```python
from build123d import *

# Parameters (mm, degrees)
SKETCH_1_W                 = 5.6
SKETCH_1_H                 = 4.2
EXTRUDE_1_DEPTH            = 1.4
SKETCH_3_W                 = 25.5
SKETCH_3_H                 = 0.3
SKETCH_3_W_2               = 5.6
EXTRUDE_2_DEPTH            = 0.2
PATTERN_START              = -2.1
PATTERN_LINEAR_1_OUTLINE_W = 5.6
PATTERN_LINEAR_1_OUTLINE_H = 1.4
PATTERN_LINEAR_1_DEPTH     = 4.2
SKETCH_4_W                 = 2.9
SKETCH_4_H                 = 1.1
SKETCH_4_H_2               = 0.55
CUT_EXTRUDE_1_DEPTH        = 0.2
SKETCH_5_W                 = 0.2
SKETCH_5_H                 = 0.8
EXTRUDE_3_DEPTH            = 0.8
SKETCH_6_W                 = 0.2
SKETCH_6_H                 = 0.8
EXTRUDE_4_DEPTH            = 0.8
SKETCH_7_W                 = 32.884134448
SKETCH_7_H                 = 1
EXTRUDE_5_DEPTH            = 0.2
CUT_EXTRUDE_START          = -0.4
SKETCH_8_W                 = 4.4
SKETCH_8_H                 = 3
CUT_EXTRUDE_2_DEPTH        = 1


# Read off the part's stored shape, not the designer's step: the pattern linear step
with BuildPart() as part:
    # Sketch 1 → Extrude 1 (new body)
    with BuildSketch(Plane.XY):
        Rectangle(SKETCH_1_W, SKETCH_1_H)
    extrude(amount=EXTRUDE_1_DEPTH)

    # Sketch 3 → Extrude 2 (add)
    with BuildSketch(Plane(origin=(0, 0, 0), x_dir=(-1, 0, 0), z_dir=(0, 0, -1))):
        Polygon((-2.8, 2.1), (2.8, 2.1), (2.8, 3.3), (-28.3, 3.3), (-28.3, 2.1), align=None)
        with Locations((-15.55, 1.95)):
            Rectangle(SKETCH_3_W, SKETCH_3_H)
        with Locations((0, 1.95)):
            Rectangle(SKETCH_3_W_2, SKETCH_3_H)
    extrude(amount=-EXTRUDE_2_DEPTH)

    # Pattern Linear 1 outline → Pattern Linear 1 (add)
    with BuildSketch(Plane(origin=(0, 0, 0), x_dir=(1, 0, 0), z_dir=(0, 1, 0)).offset(PATTERN_START)):
        with Locations((8.5, -0.7)):
            Rectangle(PATTERN_LINEAR_1_OUTLINE_W, PATTERN_LINEAR_1_OUTLINE_H)
        with Locations((17, -0.7)):
            Rectangle(PATTERN_LINEAR_1_OUTLINE_W, PATTERN_LINEAR_1_OUTLINE_H)
        with Locations((25.5, -0.7)):
            Rectangle(PATTERN_LINEAR_1_OUTLINE_W, PATTERN_LINEAR_1_OUTLINE_H)
    extrude(amount=PATTERN_LINEAR_1_DEPTH)

    # Sketch 4 → Cut-Extrude 1 (cut)
    with BuildSketch(Plane(origin=(0, 0, 0), x_dir=(-1, 0, 0), z_dir=(0, 0, -1))):
        with Locations((-4.25, 1.8)):
            Rectangle(SKETCH_4_W, SKETCH_4_H)
        with Locations((-12.75, 1.8)):
            Rectangle(SKETCH_4_W, SKETCH_4_H)
        with Locations((-21.25, 1.525)):
            Rectangle(SKETCH_4_W, SKETCH_4_H_2)
        with Locations((-21.25, 2.075)):
            Rectangle(SKETCH_4_W, SKETCH_4_H_2)
    extrude(amount=-CUT_EXTRUDE_1_DEPTH, mode=Mode.SUBTRACT)

    # Sketch 5 → Extrude 3 (add)
    with BuildSketch(Plane(origin=(28.3, 0, 0), x_dir=(0, 0, -1), z_dir=(1, 0, 0))):
        with Locations((-0.1, 2.9)):
            Rectangle(SKETCH_5_W, SKETCH_5_H)
    extrude(amount=EXTRUDE_3_DEPTH)

    # Sketch 6 → Extrude 4 (add)
    with BuildSketch(Plane.ZY.offset(2.8)):
        with Locations((0.1, 2.9)):
            Rectangle(SKETCH_6_W, SKETCH_6_H)
    extrude(amount=EXTRUDE_4_DEPTH)

    # Sketch 7 → Extrude 5 (add)
    with BuildSketch(Plane(origin=(0, 0, 0), x_dir=(-1, 0, 0), z_dir=(0, 0, -1))):
        with Locations((-12.798406479, -1.6)):
            Rectangle(SKETCH_7_W, SKETCH_7_H)
    extrude(amount=-EXTRUDE_5_DEPTH)

    # Sketch 8 → Cut-Extrude 2 (cut)
    with BuildSketch(Plane.XY.offset(1.4).offset(CUT_EXTRUDE_START)):
        Rectangle(SKETCH_8_W, SKETCH_8_H)
        with Locations((8.5, 0)):
            Rectangle(SKETCH_8_W, SKETCH_8_H)
        with Locations((17, 0)):
            Rectangle(SKETCH_8_W, SKETCH_8_H)
        with Locations((25.5, 0)):
            Rectangle(SKETCH_8_W, SKETCH_8_H)
    extrude(amount=-CUT_EXTRUDE_2_DEPTH, mode=Mode.SUBTRACT)


solid = part.part
```
Source: CAD feature listing. Evaluate the final solid. Frame: model axes, mm. A direction names the side the tool comes from. Coordinates: 2 decimals unless noted, no trailing zeros. Loops run counter-clockwise (first coordinate to the right, second up) from the corner with the lowest first, then second, coordinate; pieces in that order, holes last. Notation, with made-up numbers: M -27.75,46 L 10.25,46 A15 cw 10.25,66 Z; hole C 76.25,39 d5. An arc over 180 degrees is marked long. Put each result on its own line as item: value. Start each with the question number.
1) Cut plane C-C on x = 5. Return the cut outline in (y, z), then the cut area to 3 significant figures.
2) Cut plane D-D on x = 25.5. Return the cut outline in (y, z), then the cut area to 3 significant figures.
3) Ray query, L1, parallel to X at y = 2.2, z = 0.15; L2, parallel to Y at x = 24.5, z = 0.35; L3, parallel to Y at x = -2, z = 0.15. Return the intervals inside material, ascending. Write a range as from..to.
4) Reachability of faces 4 (the face through (17, 1.5, 0.5)), 5 (the face through (25, 0, 1.4)), 6 (the face through (-3.2, -1.6, 0.2)), 7 (the face through (0, 2.1, 1)) from +Z, -Z, +X, -X, +Y, -Y: full face, straight path, thin tool, end or side. Return the list, or none.
5) Cut plane A-A on y = 0.8. Give the number of separate pieces and of enclosed holes in the cut face, then the cut area to 3 significant figures.
6) Pull-direction query (X, two-part tool) for faces 1 (the face through (2.8, 0, 1)), 2 (the face through (17, 2.1, 1)), 3 (the face through (17, 0, 1)); classes: pulls with the +X half, pulls with the -X half, needs draft (parallel to the pull), parting line crosses it, or undercut.
7) Contact query for flat-ended pins moving along their axis: pin 1 Ø0.5 at (x, y) = (21, -1.5) entering from +Z; pin 2 Ø0.7 at (y, z) = (0, 1) entering from -X; pin 3 Ø0.7 at (y, z) = (1, 0.5) entering from +X; pin 4 Ø0.8 at (x, y) = (28.5, -1.5) entering from +Z. Output: stop coordinate, or through.
The answers:
1. outline: M -2.1,0 L -1.1,0 L -1.1,0.2 L -2.1,0.2 Z; M 2.35,0 L 3.3,0 L 3.3,0.2 L 2.35,0.2 Z
1. area: 0.390 mm²
2. outline: M -2.1,0 L -1.5,0 L -1.5,1 L 1.5,1 L 1.5,0 L 3.3,0 L 3.3,0.2 L 2.1,0.2 L 2.1,1.4 L -2.1,1.4 Z
2. area: 3.12 mm²
3. L1: x = -2.8..2.8, 5.7..11.3, 14.2..19.8, 22.7..28.3
3. L2: y = -2.1..-1.5, 1.5..2.1
3. L3: y = -2.1..-1.5, 1.5..3.3
4. face 4: -Z
4. face 5: +Z, +X, -X, +Y, -Y
4. face 6: +Z, -X, +Y, -Y
4. face 7: +Z, +X, -X, +Y
5. separate pieces: 4
5. enclosed holes: 0
5. area: 13.8 mm²
6. face 1: undercut
6. face 2: needs draft
6. face 3: undercut
7. pin 1: stops at z = 0.2
7. pin 2: stops at x = -2.8
7. pin 3: stops at x = 28.3
7. pin 4: stops at z = 1.4
